Work out the finished part from the listing and answer in its coordinate system (mm). A direction names the side the tool comes from. Coordinates: 2 decimals unless noted, no trailing zeros. Loops run counter-clockwise (first coordinate to the right, second up) from the corner with the lowest first, then second, coordinate; pieces in that order, holes last. Notation, with made-up numbers: (49, 14.25) -> (64, 14.25) arc R22 cw to (64, 53.25) -> close; hole circle Ø2 at (10.25, -4.5). An arc over 180 degrees is marked (long way). Use a Markdown table: item, result. Add a question column.
```python
from build123d import *

# Parameters (mm, degrees)
SKETCH2_R           = 8.25
BOSS_EXTRUDE1_DEPTH = 9
SKETCH3_R           = 3.175
CUT_EXTRUDE1_DEPTH  = 51
SKETCH4_OUTSIDE_W   = 22.196
SKETCH4_OUTSIDE_H   = 36.696
SKETCH4_OUTSIDE_R   = 8.25
CUT_EXTRUDE2_DEPTH  = 6
CUT_EXTRUDE3_DEPTH  = 6


with BuildPart() as part:
    # Sketch2 → Boss-Extrude1 (new body)
    with BuildSketch(Plane.XY):
        with BuildLine():
            Line((-25, 12), (25, 12))
            Line((25, 12), (25, 6))
            Line((25, 6), (22, 6))
            Line((22, 6), (22, 7))
            Line((22, 7), (16, 7))
            Line((16, 7), (16, 6))
            Line((16, 6), (14.186260959, 6))
            ThreePointArc((14.186260959, 6), (11.855802961, 4.88917059), (11.251172485, 2.379310345))
            ThreePointArc((11.251172485, 2.379310345), (0, -11.5), (-11.251172485, 2.379310345))
            ThreePointArc((-11.251172485, 2.379310345), (-11.855802961, 4.88917059), (-14.186260959, 6))
            Line((-14.186260959, 6), (-16, 6))
            Line((-16, 6), (-16, 7))
            Line((-16, 7), (-22, 7))
            Line((-22, 7), (-22, 6))
            Line((-22, 6), (-25, 6))
            Line((-25, 6), (-25, 12))
        make_face()
        Circle(SKETCH2_R, mode=Mode.SUBTRACT)
    extrude(amount=BOSS_EXTRUDE1_DEPTH)

    # Sketch3 → Cut-Extrude1 (cut, through all)
    with BuildSketch(Plane(origin=(25, 0, 0), x_dir=(0, 0, -1), z_dir=(1, 0, 0))):
        with Locations((-4.5, 13.25)):
            Circle(SKETCH3_R)
    extrude(amount=-CUT_EXTRUDE1_DEPTH, mode=Mode.SUBTRACT)

    # Sketch4 outside → Cut-Extrude2 (cut)
    with BuildSketch(Plane(origin=(-22, 0, 0), x_dir=(0, 0, -1), z_dir=(1, 0, 0))):
        with Locations((-4.5, 0.25)):
            Rectangle(SKETCH4_OUTSIDE_W, SKETCH4_OUTSIDE_H)
        with Locations((-4.5, 15.25)):
            Circle(SKETCH4_OUTSIDE_R, mode=Mode.SUBTRACT)
    extrude(amount=CUT_EXTRUDE2_DEPTH, mode=Mode.SUBTRACT)

    # Sketch5 → Cut-Extrude3 (cut)
    with BuildSketch(Plane.ZY.offset(-16)):
        with BuildLine():
            Line((0, 8.335341657), (0, 6))
            Line((0, 6), (9, 6))
            Line((9, 6), (9, 8.335341657))
            ThreePointArc((9, 8.335341657), (4.5, 7), (0, 8.335341657))
        make_face()
    extrude(amount=-CUT_EXTRUDE3_DEPTH, mode=Mode.SUBTRACT)

    # Sketch6 → Cut-Revolve1 (revolve, cut)
    with BuildSketch(Plane(origin=(0, 0, 0), x_dir=(0, 0, -1), z_dir=(1, 0, 0)), mode=Mode.PRIVATE) as cut_revolve1_sk:
        with BuildLine():
            Line((-9, 9), (-9, 0))
            Line((-9, 0), (0, 0))
            Line((0, 0), (0, 9))
            ThreePointArc((0, 9), (-4.5, 8.25), (-9, 9))
        make_face()
    revolve(cut_revolve1_sk.sketch.rotate(Axis((0, 0, 9), (0, 0, 1)), 90), axis=Axis((0, 0, 9), (0, 0, 1)), mode=Mode.SUBTRACT)  # turned: the seam where the file's is


solid = part.part
```
Item 1: Section C-C (z = 4.25) is taken. Determine the outline of the cut face in (x, y), then the cut area to 3 significant figures.
Item 2: Section B-B (x = 0) is taken. Determine the outline of the cut face in (y, z) (3 decimals).
Item 3: Find the intervals of material crossed by probe 1 along X at (y, z) = (6.25, 4); probe 2 along X at (y, z) = (6.5, 8.5); probe 3 along X at (y, z) = (-0.75, 5), in increasing order.
Item 4: For faces 4 (the face through (0, 12, 1)), 5 (the face through (-23, 6, 4)), 6 (the face through (15, 6, 4)), 7 (the face through (19, 7, 4.6)), 8 (the face through (11.88, 4.92, 4.44)), determine the directions among +Z, -Z, +X, -X, +Y, -Y from which every point of the face is accessible in a straight line to the end or side of a thin tool.
Item 5: Given pin 1 (2.5 mm diameter, centred on x = -23, z = 6.5, fed in from -Y); pin 2 (1.5 mm diameter, centred on x = -14.5, y = 5, fed in from -Z); pin 3 (1.5 mm diameter, centred on x = 18, z = 2, fed in from -Y); pin 4 (1.5 mm diameter, centred on x = -13, z = 7.5, fed in from -Y), each flat-ended and moving along its own axis, determine where each tip first touches the part or whether it passes through.
Item 6: For a pull along X with two mould halves and no side action, classify faces 1 (the face through (-19, 7, 4.4)), 2 (the face through (0.35, 10.075, 4.552)), 3 (the face through (-11.83, 4.86, 4.44)) as +X half, -X half, draft (parallel to the pull), parting line (faces both ways), or undercut.
Item 7: Section A-A (y = 0) is taken. Determine the outline of the cut face in (x, z) (3 decimals), then the cut area to 3 significant figures.
Item 8: Section D-D (z = 2.25) is taken. Determine the outline of the cut face in (x, y), then the cut area to 3 significant figures.
Output:
| question | item | result |
|---|---|---|
| 1 | outline | (-25, 6) -> (-22, 6) -> (-22, 7) -> (-16, 7) -> (-16, 6) -> (-14.19, 6) arc R3 cw to (-11.25, 2.38) arc R11.5 ccw (long way) to (11.25, 2.38) arc R3 cw to (14.19, 6) -> (16, 6) -> (16, 7) -> (22, 7) -> (22, 6) -> (25, 6) -> (25, 10.08) -> (-25, 10.08) -> close; hole circle Ø16.5 at (0, 0) |
| 1 | area | 325 mm2 |
| 2 | outline | (-11.5, 0) -> (-9, 0) arc R13.875 ccw to (-9, 9) -> (-11.5, 9) -> close; (9, 0) -> (12, 0) -> (12, 1.581) arc R3.175 cw to (12, 7.419) -> (12, 9) -> (9, 9) arc R13.875 ccw to start |
| 3 | probe 1 | x = -25 to -22, -16 to -5.4, 5.4 to 16, 22 to 25 |
| 3 | probe 2 | x = -25 to -22, -16 to -5.99, 5.99 to 16, 22 to 25 |
| 3 | probe 3 | x = -11.48 to -8.22, 8.22 to 11.48 |
| 4 | face 4 | +Z, -Z, +X, -X, +Y |
| 4 | face 5 | +Z, -Z, -X, -Y |
| 4 | face 6 | +Z, -Z, +X, -Y |
| 4 | face 7 | -Y |
| 4 | face 8 | +Z, -Z, +X |
| 5 | pin 1 | stops at y = 6 |
| 5 | pin 2 | passes through |
| 5 | pin 3 | stops at y = 7.19 |
| 5 | pin 4 | stops at y = 5.29 |
| 6 | face 1 | undercut |
| 6 | face 2 | draft |
| 6 | face 3 | -X half |
| 7 | outline | (-11.5, 0) -> (-9, 0) arc R13.875 ccw to (-9, 9) -> (-11.5, 9) -> close; (9, 0) -> (11.5, 0) -> (11.5, 9) -> (9, 9) arc R13.875 ccw to start |
| 7 | area | 54.0 mm2 |
| 8 | outline | (-25, 6) -> (-22, 6) -> (-22, 7.31) -> (-16, 7.31) -> (-16, 6) -> (-14.19, 6) arc R3 cw to (-11.25, 2.38) arc R11.5 ccw (long way) to (11.25, 2.38) arc R3 cw to (14.19, 6) -> (16, 6) -> (16, 7.31) -> (22, 7.31) -> (22, 6) -> (25, 6) -> (25, 11.01) -> (-25, 11.01) -> close; hole circle Ø16.87 at (0, 0) |
| 8 | area | 358 mm2 |
